from build123d import *

# Parameters (mm, degrees)
BOSS_EXTRU_1_DEPTH      = 45
ENL_V_MAT_EXTRU_1_DEPTH = 43
ENL_V_MAT_EXTRU_2_DEPTH = 95.855152733
CHANFREIN1_SIZE         = 1
ESQUISSE6_W             = 10
ESQUISSE6_H             = 15
ESQUISSE6_W_2           = 4
ESQUISSE6_H_2           = 9
BOSS_EXTRU_2_DEPTH      = 5
ESQUISSE8_W             = 11
ESQUISSE8_H             = 8
ENL_V_MAT_EXTRU_5_DEPTH = 10


with BuildPart() as part:
    # Esquisse1 → Boss.-Extru.1 (new body)
    with BuildSketch(Plane.XY):
        with BuildLine():
            Line((6, 0), (44.5, 0))
            ThreePointArc((44.5, 0), (48.742640687, 1.757359313), (50.5, 6))
            Line((50.5, 6), (50.5, 60.5))
            ThreePointArc((50.5, 60.5), (48.742640687, 64.742640687), (44.5, 66.5))
            Line((44.5, 66.5), (6, 66.5))
            ThreePointArc((6, 66.5), (1.757359313, 64.742640687), (0, 60.5))
            Line((0, 60.5), (0, 6))
            ThreePointArc((0, 6), (1.757359313, 1.757359313), (6, 0))
        make_face()
    extrude(amount=BOSS_EXTRU_1_DEPTH)

    # Esquisse3 → Enlèv. mat.-Extru.1 (cut)
    with BuildSketch(Plane.XY.offset(45)):
        with BuildLine():
            Line((2, 60.5), (2, 6))
            ThreePointArc((2, 6), (3.171572875, 3.171572875), (6, 2))
            Line((6, 2), (44.5, 2))
            ThreePointArc((44.5, 2), (47.328427125, 3.171572875), (48.5, 6))
            Line((48.5, 6), (48.5, 60.5))
            ThreePointArc((48.5, 60.5), (47.328427125, 63.328427125), (44.5, 64.5))
            Line((44.5, 64.5), (6, 64.5))
            ThreePointArc((6, 64.5), (3.171572875, 63.328427125), (2, 60.5))
        make_face()
    extrude(amount=-ENL_V_MAT_EXTRU_1_DEPTH, mode=Mode.SUBTRACT)

    # Esquisse4 → Enlèv. mat.-Extru.2 (cut, through all)
    with BuildSketch(Plane(origin=(50.5, 0, 0), x_dir=(0, 0, -1), z_dir=(1, 0, 0))):
        with BuildLine():
            Line((-57.973811458, 63), (-3.5, 63))
            ThreePointArc((-3.5, 63), (-2.792893219, 62.707106781), (-2.5, 62))
            Line((-2.5, 62), (-2.5, 55))
            ThreePointArc((-2.5, 55), (-2.792893219, 54.292893219), (-3.5, 54))
            Line((-3.5, 54), (-57.973811458, 54))
            Line((-57.973811458, 54), (-57.973811458, 63))
        make_face()
    extrude(amount=-ENL_V_MAT_EXTRU_2_DEPTH, mode=Mode.SUBTRACT)

    # Chanfrein1
    chanfrein1_edges = [part.edges().sort_by_distance(p)[0] for p in [
        (50.5, 33.25, 0),
        (48.742640687, 1.757359313, 0),
        (25.25, 0, 0),
        (1.757359313, 1.757359313, 0),
        (0, 33.25, 0),
        (1.757359313, 64.742640687, 0),
        (25.25, 66.5, 0),
        (48.742640687, 64.742640687, 0),
    ]]
    chamfer(chanfrein1_edges, length=CHANFREIN1_SIZE)

    # Esquisse6 → Boss.-Extru.2 (add)
    with BuildSketch(Plane.XY.offset(2)):
        with Locations((26.5, 36.5)):
            Rectangle(ESQUISSE6_W, ESQUISSE6_H)
        with Locations((26.5, 36.5)):
            Rectangle(ESQUISSE6_W_2, ESQUISSE6_H_2, mode=Mode.SUBTRACT)
    extrude(amount=BOSS_EXTRU_2_DEPTH)

    # Esquisse8 → Enlèv. mat.-Extru.5 (cut)
    with BuildSketch(Plane.XZ):
        with Locations((24.25, 14)):
            Rectangle(ESQUISSE8_W, ESQUISSE8_H)
    extrude(amount=-ENL_V_MAT_EXTRU_5_DEPTH, mode=Mode.SUBTRACT)


solid = part.part
The listing builds one solid part. Answer for the finished solid, in the listing's coordinates (mm). A direction names the side the tool comes from. Give positions to 0.01 mm unless a question says otherwise; leave off trailing zeros. Order: outer loops, then holes, each group sorted by start corner. A loop starts at its lowest first (then second) coordinate and runs counter-clockwise, first axis right, second up. Notation, with made-up numbers: (-21.75, 32) - (1.25, 32) arc R11 ccw to (1.25, 49) - close; hole circle Ø10 at (81, -23). An arc over 180 degrees is marked (long way). Use one line per item in the form item = value.
1) Find section A-A on z = 29.5. Determine the outline of the cut face in (x, y), and give its area (3 significant figures).
Verdict:
outline = (0, 6) arc R6 ccw to (6, 0) - (44.5, 0) arc R6 ccw to (50.5, 6) - (50.5, 54) - (48.5, 54) - (48.5, 6) arc R4 cw to (44.5, 2) - (6, 2) arc R4 cw to (2, 6) - (2, 54) - (0, 54) - close; (0.55, 63) - (2.88, 63) arc R4 cw to (6, 64.5) - (44.5, 64.5) arc R4 cw to (47.62, 63) - (49.95, 63) arc R6 ccw to (44.5, 66.5) - (6, 66.5) arc R6 ccw to start
area = 398 mm^2
2) Each of these flat-tipped pins is pushed along its axis until it touches: pin 1 (3 mm diameter, centred on x = 25.5, y = 37.5, fed in from +Z); pin 2 (2 mm diameter, centred on y = 0.5, z = 13, fed in from -X); pin 3 (2 mm diameter, centred on y = 1, z = 13, fed in from +X). Where does it stop, or does it pass through?
Verdict:
pin_1 = 7
pin_2 = 2.03
pin_3 = 48.97
3) The mould has two halves that part along X. Classify faces 1 (the flat face through (28.5, 36, 4)), 2 (the flat face through (26, 64.5, 24)), 3 (the flat face through (49, 63, 25)), 4 (the flat face through (0, 34, 23)): released by +X, released by -X, zero draft, split by the parting line, or undercut.
Verdict:
face_1 = undercut
face_2 = undercut
face_3 = zero draft
face_4 = released by -X
4) Find section B-B on x = 27. Determine the outline of the cut face in (y, z).
Verdict:
outline = (0, 1) - (1, 0) - (65.5, 0) - (66.5, 1) - (66.5, 45) - (64.5, 45) - (64.5, 2) - (44, 2) - (44, 7) - (41, 7) - (41, 2) - (32, 2) - (32, 7) - (29, 7) - (29, 2) - (2, 2) - (2, 10) - (0, 10) - close; (0, 18) - (2, 18) - (2, 45) - (0, 45) - close
5) Find section C-C on y = 38.5. Determine the outline of the cut face in (x, z), and give its area (3 significant figures).
Verdict:
outline = (0, 1) - (1, 0) - (49.5, 0) - (50.5, 1) - (50.5, 45) - (48.5, 45) - (48.5, 2) - (31.5, 2) - (31.5, 7) - (28.5, 7) - (28.5, 2) - (24.5, 2) - (24.5, 7) - (21.5, 7) - (21.5, 2) - (2, 2) - (2, 45) - (0, 45) - close
area = 302 mm^2
6) For faces 5 (the flat face through (24.5, 36, 4)), 6 (the flat face through (2, 63, 25)), 7 (the flat face through (29.75, 1, 14)), 8 (the flat face through (25, 65, 45)), determine the directions among +Z, -Z, +X, -X, +Y, -Y from which every point of the face is accessible in a straight line to the end or side of a thin tool.
Verdict:
face_5 = +Z
face_6 = +Z, +X, -X
face_7 = -Y
face_8 = +Z, +X, -X, +Y, -Y
7) Find section D-D on x = 17. Determine the outline of the cut face in (y, z), and give its area (3 significant figures).
Verdict:
outline = (0, 1) - (1, 0) - (65.5, 0) - (66.5, 1) - (66.5, 45) - (64.5, 45) - (64.5, 2) - (2, 2) - (2, 45) - (0, 45) - close
area = 304 mm^2
8) Consider probe 1 along Y at (x, z) = (10, 30); probe 2 along X at (y, z) = (22, 36.5); probe 3 along Y at (x, z) = (47, 9). Determine where each line is inside the solid, lowest interval first. Write a range as [from, to].
Verdict:
probe_1 = [0, 2], [64.5, 66.5]
probe_2 = [0, 2], [48.5, 50.5]
probe_3 = [0.55, 2.88], [63.62, 65.95]
